Can you work these out from the model? Positions are in its coordinate system, mm. A direction names the side the tool comes from. Give positions to 0.01 mm unless a question says otherwise; leave off trailing zeros. Loops run counter-clockwise (first coordinate to the right, second up) from the corner with the lowest first, then second, coordinate; pieces in that order, holes last. Notation, with made-up numbers: (78, -28) - (87, -28) arc R26 ccw to (87, -9) - close; hole circle Ø10 at (33, 0.5). An arc over 180 degrees is marked (long way). Answer as a JSON object with one key per item and string values.
```python
from build123d import *

# Parameters (mm, degrees)
F2_R     = 4.7625
F3_DEPTH = 9.525


# Not quite as in the source:
# - the program builds the solid bodies; features that only make, move or delete a surface that nothing else refers to are left out


with BuildPart() as f1:
    # F0 (on Front) → F1 (revolve)
    with BuildSketch(Plane.XZ):
        Polygon((0, 63.5), (0, 0), (88.9, 39.4620286852), (88.9, 50.8), (25.4, 50.8), (25.4, 63.5), align=None)
    revolve(axis=Axis((0, 0, 31.75), (0, 0, -1)))

    # F2 (on face) → F3 (cut)
    with BuildSketch(Plane.XY.offset(63.5)):
        Circle(F2_R)
    extrude(amount=-F3_DEPTH, mode=Mode.SUBTRACT)


solid = f1.part
```
1) I'm going to push flat-ended pins straight in: P1, Ø1.5, axis at x = 68.5, z = 53, coming from the -Y side; P2, Ø3, axis at x = -10.5, y = -28, coming from the -Z side; P3, Ø3, axis at x = 0.5, y = -61.5, coming from the +Z side; P4, Ø5, axis at y = 1, z = 22.5, coming from the -X side. Where does each tip first touch, or does it pass through?
Check sheet entries:
{"P1": "through", "P2": "z = 12.61", "P3": "z = 50.8", "P4": "x = -56.31"}
2) Imagine slicing it at A-A on z = 47. Write out the boundary of the cut face in (x, y), and give its area (3 significant figures).
Check sheet entries:
{"outline": "circle Ø177.8 at (0, 0)", "area": "24,800 mm2"}
3) If we mould it in two halves opening along X, with no side actions, what happens to faces 1 (the cylindrical face through (-3.78, -2.9, 58.8)), 2 (the conical face through (-1.21, 5.43, 2.47)), 3 (the flat face through (5, 0, 63.5))? For each: released by +X, released by -X, zero draft, split by the parting line, or undercut.
Check sheet entries:
{"face 1": "undercut", "face 2": "split by the parting line", "face 3": "zero draft"}
4) Imagine slicing it at B-B on z = 12. Write out the boundary of the cut face in (x, y), and give its area (3 significant figures).
Check sheet entries:
{"outline": "circle Ø54.07 at (0, 0)", "area": "2,300 mm2"}
5) Which directions (+Z, -Z, +X, -X, +Y, -Y) give clear straight access to the entire face, cutting with the end or side of a thin tool? Please do faces 4 (the flat face through (19, 19, 50.8)), 5 (the cylindrical face through (84.795, -26.703, 45.21)).
Check sheet entries:
{"face 4": "+Z", "face 5": "+Z, -Z"}
6) I need wall thicknesses on L1, parallel to Y at x = 0, z = 61.75; L2, parallel to Z at x = 2.5, y = 15; L3, parallel to Z at x = -65, y = 8. Which ranges of each line are inside material? Lowest first, please.
Check sheet entries:
{"L1": "-25.4 to -4.76, 4.76 to 25.4", "L2": "6.75 to 63.5", "L3": "29.07 to 50.8"}
